The figure shows three views and two pictorial views of one solid part (mm, origin at its lowest corner). Answer the questions. A direction names the side the tool comes from. Give positions to 0.01 mm unless a question says otherwise; leave off trailing zeros. Order: outer loops, then holes, each group sorted by start corner. A loop starts at its lowest first (then second) coordinate and runs counter-clockwise, first axis right, second up. Notation, with made-up numbers: (86, 84.5) - (124, 84.5) arc R20 cw to (124, 111.5) - close; hole circle Ø10 at (74, 86.5). An arc over 180 degrees is marked (long way). Use a Markdown table: item, result. Add a question column.
1. A cutting plane is placed at D-D on y = 716. Determine the outline of the cut face in (x, z).
2. Consider L1, parallel to Z at x = 350, y = 705; L2, parallel to X at y = 386.5, z = 193.5; L3, parallel to Y at x = 126, z = 227.5. Determine where each line is inside the solid, lowest interval first.
3. For a pull along X with two mould halves and no side action, classify the marked faces 1, 2, 3 and 4 as released by +X, released by -X, zero draft, split by the parting line, or undercut.
4. Flat-ended cylindrical pins translate along their axes: P1, Ø3, axis at x = 111, z = 253, coming from the +Y side; P2, Ø6, axis at x = 203.5, z = 73, coming from the -Y side. Find the tip coordinate at first contact, or state that the pin passes through.
5. A cutting plane is placed at A-A on y = 466. Determine the outline of the cut face in (x, z), and give its area (3 significant figures).
6. A cutting plane is placed at B-B on z = 150. Determine the outline of the cut face in (x, y), and give its area (3 significant figures).
7. A cutting plane is placed at C-C on x = 180. Determine the outline of the cut face in (y, z).
8. Which of the six approach directions +Z, -Z, +X, -X, +Y, -Y give full straight-line access (tool end or side, diameter ignored) to the marked faces 5, 6 and 7?
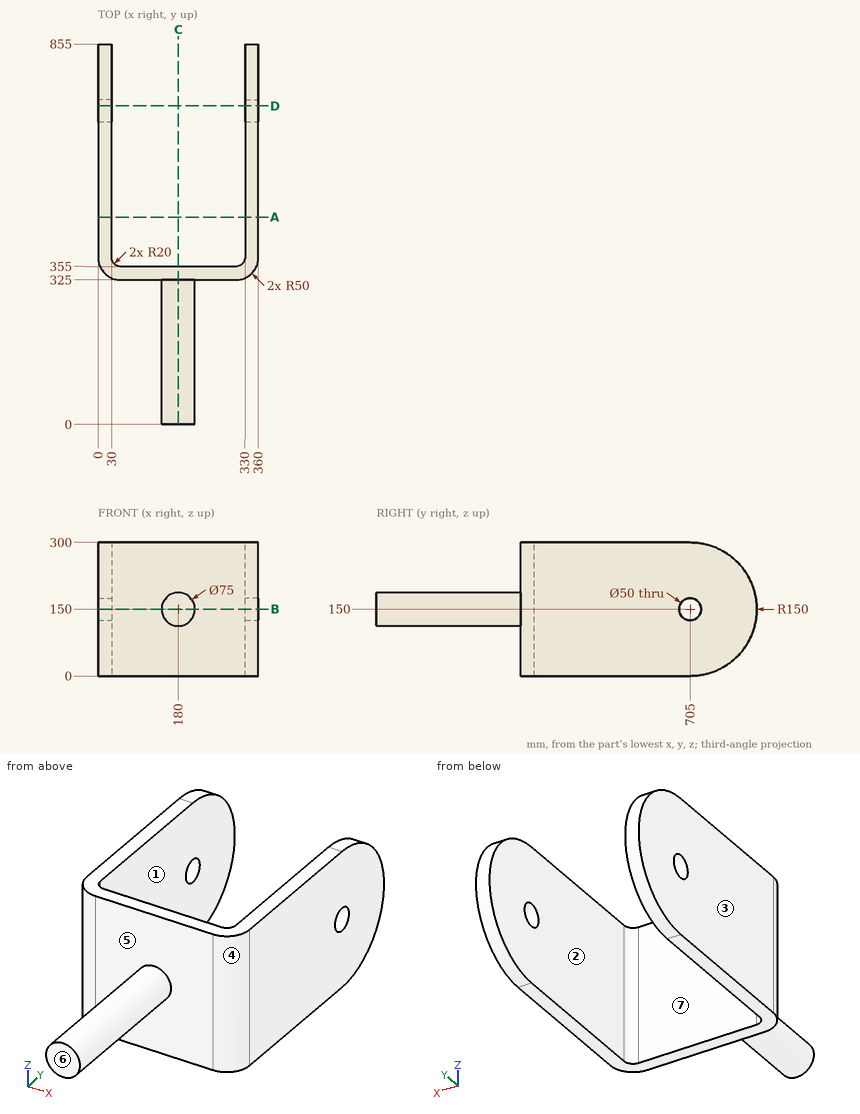
Output values:
| question | item | result |
|---|---|---|
| 1 | outline | (0, 0.4) - (30, 0.4) - (30, 127.55) - (0, 127.55) - close; (0, 172.45) - (30, 172.45) - (30, 299.6) - (0, 299.6) - close; (330, 0.4) - (360, 0.4) - (360, 127.55) - (330, 127.55) - close; (330, 172.45) - (360, 172.45) - (360, 299.6) - (330, 299.6) - close |
| 2 | L1 | 0 to 125, 175 to 300 |
| 2 | L2 | 0 to 30, 330 to 360 |
| 2 | L3 | 325 to 355 |
| 3 | face 1 | undercut |
| 3 | face 2 | undercut |
| 3 | face 3 | released by -X |
| 3 | face 4 | released by +X |
| 4 | P1 | y = 355 |
| 4 | P2 | y = 325 |
| 5 | outline | (0, 0) - (30, 0) - (30, 300) - (0, 300) - close; (330, 0) - (360, 0) - (360, 300) - (330, 300) - close |
| 5 | area | 18,000 mm² |
| 6 | outline | (0, 375) arc R50 ccw to (50, 325) - (142.5, 325) - (142.5, 0) - (217.5, 0) - (217.5, 325) - (310, 325) arc R50 ccw to (360, 375) - (360, 680) - (330, 680) - (330, 375) arc R20 cw to (310, 355) - (50, 355) arc R20 cw to (30, 375) - (30, 680) - (0, 680) - close; (0, 730) - (30, 730) - (30, 855) - (0, 855) - close; (330, 730) - (360, 730) - (360, 855) - (330, 855) - close |
| 6 | area | 61,300 mm² |
| 7 | outline | (0, 112.5) - (325, 112.5) - (325, 0) - (355, 0) - (355, 300) - (325, 300) - (325, 187.5) - (0, 187.5) - close |
| 8 | face 5 | -Y |
| 8 | face 6 | +Z, -Z, +X, -X, -Y |
| 8 | face 7 | +Z, -Z, +Y |
